from build123d import *

# Parameters (mm, degrees)
SZKIC1_R                         = 14.5
SZKIC1_R_2                       = 5
DODANIE_WYCI_GNI_CIE1_DEPTH      = 15
OTW_R_GWINTOWANY_M61_D           = 5
WYTNIJ_WYCI_GNI_CIE2_DEPTH       = 10
WYTNIJ_WYCI_GNI_CIE4_START       = 20
WYTNIJ_WYCI_GNI_CIE4_DEPTH       = 20
SFAZOWANIE4_SIZE                 = 10
SZKIC17_R                        = 7.5
WYTNIJ_WYCI_GNI_CIE5_DEPTH       = 5
SZKIC17_5_R                      = 7.5
WYTNIJ_WYCI_GNI_CIE6_DEPTH       = 163.311542951
OTW_R_GWINTOWANY_M81_D           = 6.8
OTW_R_GWINTOWANY_M81_DEPTH       = 16.207073895
OTW_R_GWINTOWANY_M81_CSINK_D     = 8.05
OTW_R_GWINTOWANY_M81_CSINK_ANGLE = 90
OTW_R_GWINTOWANY_M81_TIP         = 2.042926105


with BuildPart() as part:
    # Szkic1 → Dodanie-wyci_gni_cie1 (new, symmetric)
    with BuildSketch(Plane(origin=(0, 0, 0), x_dir=(0, 0, -1), z_dir=(1, 0, 0))):
        with BuildLine():
            Line((-72.530533194, -70), (-85.848604083, -57.040111879))
            ThreePointArc((-85.848604083, -57.040111879), (-92.404294481, -44.130927243), (-87.495806927, -30.50995538))
            ThreePointArc((-87.495806927, -30.50995538), (-75.419960244, 0), (-87.495806927, 30.50995538))
            ThreePointArc((-87.495806927, 30.50995538), (-92.32041193, 40.919666146), (-89.978943384, 52.151603499))
            ThreePointArc((-89.978943384, 52.151603499), (-81.115709466, 65.086416999), (-70.408575711, 76.541704099))
            ThreePointArc((-70.408575711, 76.541704099), (-67.080888035, 80.867469231), (-65.40069858, 86.060032436))
            Line((-65.40069858, 86.060032436), (-62.076569761, 109.385977671))
            ThreePointArc((-62.076569761, 109.385977671), (-54.044566654, 124.12820267), (-38.316621209, 130))
            Line((-38.316621209, 130), (38.316621209, 130))
            ThreePointArc((38.316621209, 130), (54.044566654, 124.12820267), (62.076569761, 109.385977671))
            Line((62.076569761, 109.385977671), (65.40069858, 86.060032436))
            ThreePointArc((65.40069858, 86.060032436), (67.080888035, 80.867469231), (70.408575711, 76.541704099))
            ThreePointArc((70.408575711, 76.541704099), (81.115709466, 65.086416999), (89.978943384, 52.151603499))
            ThreePointArc((89.978943384, 52.151603499), (92.32041193, 40.919666146), (87.495806927, 30.50995538))
            ThreePointArc((87.495806927, 30.50995538), (75.419960244, 0), (87.495806927, -30.50995538))
            ThreePointArc((87.495806927, -30.50995538), (92.006314233, -46.663708643), (81.240664282, -59.524081957))
            Line((81.240664282, -59.524081957), (51.469466806, -70))
            Line((51.469466806, -70), (51.469466806, -100))
            ThreePointArc((51.469466806, -100), (48.29757558, -114.988630917), (39.325734007, -127.407407407))
            ThreePointArc((39.325734007, -127.407407407), (36.208235452, -129.329364235), (32.607823953, -130))
            Line((32.607823953, -130), (14.469466806, -130))
            Line((14.469466806, -130), (-35.530533194, -130))
            Line((-35.530533194, -130), (-53.668890342, -130))
            ThreePointArc((-53.668890342, -130), (-57.269301841, -129.329364235), (-60.386800396, -127.407407407))
            ThreePointArc((-60.386800396, -127.407407407), (-69.358641969, -114.988630917), (-72.530533194, -100))
            Line((-72.530533194, -100), (-72.530533194, -70))
        make_face()
        Circle(SZKIC1_R, mode=Mode.SUBTRACT)
        with Locations(Location((74.189369185, -43, 0), (0, 0, 180))):
            Circle(SZKIC1_R_2, mode=Mode.SUBTRACT)
        with Locations(Location((74.189369185, 43, 0), (0, 0, 180))):
            Circle(SZKIC1_R_2, mode=Mode.SUBTRACT)
        with BuildLine():
            Line((14.469466806, -84), (-35.530533194, -84))
            ThreePointArc((-35.530533194, -84), (-51.530533194, -100), (-35.530533194, -116))
            Line((-35.530533194, -116), (14.469466806, -116))
            ThreePointArc((14.469466806, -116), (30.469466806, -100), (14.469466806, -84))
        make_face(mode=Mode.SUBTRACT)
    extrude(amount=DODANIE_WYCI_GNI_CIE1_DEPTH, both=True)

    # Otw_r gwintowany M61 (through all)
    with Locations(Plane(origin=(-15, 0, 0), x_dir=(0, 0, -1), z_dir=(-1, 0, 0))):
        with Locations((-29.434757864, -101.542610293), (50.455604917, -97.355733794)):
            Hole(OTW_R_GWINTOWANY_M61_D / 2)

    # Szkic12 → Wytnij-wyci_gni_cie2 (cut)
    with BuildSketch(Plane(origin=(-15, 0, 0), x_dir=(0, 0, -1), z_dir=(1, 0, 0))):
        with BuildLine():
            Line((28.802174659, 93.483680258), (-9.732880373, 95.503216916))
            ThreePointArc((-9.732880373, 95.503216916), (-14.464348266, 100.758044371), (-9.209520811, 105.489512264))
            Line((-9.209520811, 105.489512264), (29.325534221, 103.469975605))
            ThreePointArc((29.325534221, 103.469975605), (34.057002114, 98.21514815), (28.802174659, 93.483680258))
        make_face()
    extrude(amount=WYTNIJ_WYCI_GNI_CIE2_DEPTH, mode=Mode.SUBTRACT)

    # Szkic16 → Wytnij-wyci_gni_cie4 (cut)
    with BuildSketch(Plane(origin=(-15, 0, 0), x_dir=(0, 0, -1), z_dir=(1, 0, 0)).offset(WYTNIJ_WYCI_GNI_CIE4_START)):
        with BuildLine():
            Line((-53.668890342, -130), (32.607823953, -130))
            ThreePointArc((32.607823953, -130), (36.208235452, -129.329364235), (39.325734007, -127.407407407))
            ThreePointArc((39.325734007, -127.407407407), (48.29757558, -114.988630917), (51.469466806, -100))
            Line((51.469466806, -100), (51.469466806, -70))
            Line((51.469466806, -70), (-72.530533194, -70))
            Line((-72.530533194, -70), (-72.530533194, -100))
            ThreePointArc((-72.530533194, -100), (-69.358641969, -114.988630917), (-60.386800396, -127.407407407))
            ThreePointArc((-60.386800396, -127.407407407), (-57.269301841, -129.329364235), (-53.668890342, -130))
        make_face()
        with BuildLine():
            Line((-35.530533194, -116), (14.469466806, -116))
            ThreePointArc((14.469466806, -116), (30.469466806, -100), (14.469466806, -84))
            Line((14.469466806, -84), (-35.530533194, -84))
            ThreePointArc((-35.530533194, -84), (-51.530533194, -100), (-35.530533194, -116))
        make_face(mode=Mode.SUBTRACT)
    extrude(amount=-WYTNIJ_WYCI_GNI_CIE4_DEPTH, mode=Mode.SUBTRACT)

    # Sfazowanie4
    sfazowanie4_edges = [part.edges().sort_by_distance(p)[0] for p in [
        (-15, -70, 10.530533194),
    ]]
    chamfer(sfazowanie4_edges, length=SFAZOWANIE4_SIZE)

    # Szkic17 → Wytnij-wyci_gni_cie5 (cut)
    with BuildSketch(Plane(origin=(-15, 0, 0), x_dir=(0, 0, -1), z_dir=(1, 0, 0))):
        with BuildLine():
            Line((-45.292857142, 8.957177033), (-31.578571428, 10.93666367))
            ThreePointArc((-31.578571428, 10.93666367), (-22.462605729, 8.080234378), (-18.98012619, -0.815402484))
            ThreePointArc((-18.98012619, -0.815402484), (-23.079412621, -8.614404816), (-31.578571429, -10.936663671))
            Line((-31.578571429, -10.936663671), (-45.292857143, -8.957177034))
            ThreePointArc((-45.292857143, -8.957177034), (-53.05, 0), (-45.292857142, 8.957177033))
        make_face()
        with Locations(Location((-30, -1e-09, 0), (0, 0, 180))):
            Circle(SZKIC17_R, mode=Mode.SUBTRACT)
    extrude(amount=WYTNIJ_WYCI_GNI_CIE5_DEPTH, mode=Mode.SUBTRACT)

    # Szkic17_5 → Wytnij-wyci_gni_cie6 (cut, through all)
    with BuildSketch(Plane(origin=(-15, 0, 0), x_dir=(0, 0, -1), z_dir=(1, 0, 0))):
        with Locations(Location((-30, -1e-09, 0), (0, 0, 180))):
            Circle(SZKIC17_5_R)
    extrude(amount=WYTNIJ_WYCI_GNI_CIE6_DEPTH, mode=Mode.SUBTRACT)

    # Otw_r gwintowany M81
    with Locations(Plane(origin=(5, -77, -39.469466806), x_dir=(0, 0, -1), z_dir=(-1, 0, 0))):
        with Locations((0, 0), (0, 40), (-100, 40), (-100, 0)):
            CounterSinkHole(OTW_R_GWINTOWANY_M81_D / 2, OTW_R_GWINTOWANY_M81_CSINK_D / 2, depth=OTW_R_GWINTOWANY_M81_DEPTH, counter_sink_angle=OTW_R_GWINTOWANY_M81_CSINK_ANGLE)
            with Locations((0, 0, -(OTW_R_GWINTOWANY_M81_DEPTH + OTW_R_GWINTOWANY_M81_TIP / 2))):  # 118° drill point
                Cone(0, OTW_R_GWINTOWANY_M81_D / 2, OTW_R_GWINTOWANY_M81_TIP, mode=Mode.SUBTRACT)


solid = part.part
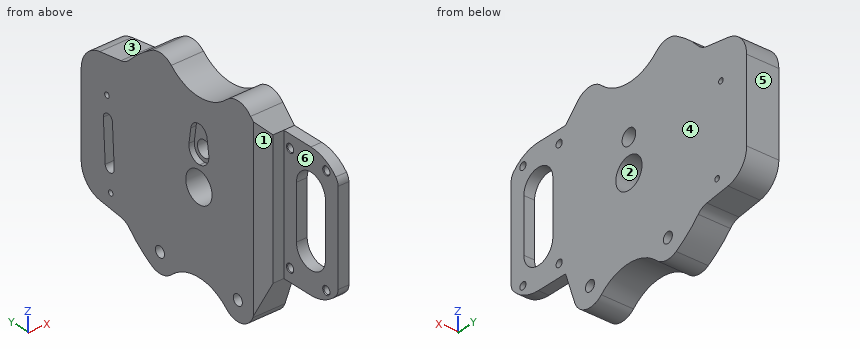
Build history of the part. All positions in model axes, mm. Face numbers are marked on the shaded views. A direction names the side the tool comes from. Round coordinates to 2 decimals unless told otherwise and drop trailing zeros. Loops run counter-clockwise (first coordinate to the right, second up) from the corner with the lowest first, then second, coordinate; pieces in that order, holes last. Notation, with made-up numbers: (83, 60) -> (87, 60) arc R14 cw to (87, 75) -> close; hole circle Ø10 at (76.5, 74). An arc over 180 degrees is marked (long way). One line per item, written item: value. Start each with the question number.
Q1. Two-plate mould, pull along Y, no slides. Class the marked faces 1, 2, 3 and 4: released by +Y, released by -Y, zero draft, split by the parting line, or undercut.
Q2. Cut at A-A on y = -77. List the corners of the cut face in (x, z) (3 decimals), plus the area to 3 significant figures.
Q3. Drop flat-ended pins along their axis: pin 1 Ø1.5 at (x, y) = (-0.5, 76) entering from +Z; pin 2 Ø11 at (y, z) = (-117, -39.47) entering from -X; pin 3 Ø10 at (y, z) = (7, 1) entering from -X; pin 4 Ø6.5 at (y, z) = (-4.5, 40.5) entering from -X. Give the stop position or say it passes through.
Q4. Cut at C-C on x = 2. List the corners of the cut face in (y, z).
Q5. Cut at D-D on z = 42.5. List the corners of the cut face in (x, y), plus the area to 3 significant figures.
Q6. 3-axis set-ups, long thin cutter, end or side, ignore diameter. For the marked faces 5 and 6: which of +Z, -Z, +X, -X, +Y, -Y reach the whole face in a straight line?
Q7. Cut at B-B on z = 0. List the corners of the cut face in (x, y), plus the area to 3 significant figures.
Q8. Probe line 1 along Z through (x, y) = (12.5, -77); line 2 along Y through (x, z) = (-4, 30); line 3 along Y through (x, z) = (-12, -84). List the from-to ranges inside material, lowest first.
Computed:
1. face 1: released by -Y
1. face 2: undercut
1. face 3: released by +Y
1. face 4: zero draft
2. outline: (5, -51.469) -> (15, -51.469) -> (15, -42.869) -> (5.625, -42.869) -> (5, -43.494) -> close; (5, -35.444) -> (5.625, -36.069) -> (15, -36.069) -> (15, 57.131) -> (5.625, 57.131) -> (5, 56.506) -> close; (5, 64.556) -> (5.625, 63.931) -> (15, 63.931) -> (15, 72.531) -> (5, 72.531) -> close
2. area: 1,100 mm²
3. pin 1: z = 71.79
3. pin 2: x = 5
3. pin 3: through
3. pin 4: x = -10
4. outline: (-70, -51.47) -> (-59.52, -81.24) arc R18 ccw to (-30.51, -87.5) arc R44.58 cw to (30.51, -87.5) arc R18.25 ccw to (52.15, -89.98) arc R104 ccw to (76.54, -70.41) arc R16 cw to (86.06, -65.4) -> (109.39, -62.08) arc R24 ccw to (130, -38.32) -> (130, 38.32) arc R24 ccw to (109.39, 62.08) -> (86.06, 65.4) arc R16 cw to (76.54, 70.41) arc R104 ccw to (52.15, 89.98) arc R18.25 ccw to (30.51, 87.5) arc R44.58 cw to (-30.51, 87.5) arc R18.25 ccw to (-57.04, 85.85) -> (-70, 72.53) -> close; hole circle Ø10 at (-43, -74.19); hole circle Ø29 at (0, 0); hole circle Ø15 at (0, 30); hole circle Ø10 at (43, -74.19); hole circle Ø5 at (97.36, -50.46); hole circle Ø5 at (101.54, 29.43)
5. outline: (-15, -60) -> (-5, -70) -> (5, -70) -> (5, -85.6) -> (15, -85.6) -> (15, 129.63) -> (-15, 129.63) -> (-15, 9.36) -> (-10, 9.36) -> (-10, -9.36) -> (-15, -9.36) -> close; (5, -130) -> (15, -130) -> (15, -114.4) -> (5, -114.4) -> close
5. area: 6,160 mm²
6. face 5: +Z, -Z, +X, -X, +Y
6. face 6: +Z, -Z, -X, -Y
7. outline: (-15, -60) -> (-5, -70) -> (5, -70) -> (5, -84) -> (15, -84) -> (15, -14.5) -> (-15, -14.5) -> close; (-15, 14.5) -> (15, 14.5) -> (15, 130) -> (-15, 130) -> (-15, 105.01) -> (-5, 105.01) -> (-5, 94.99) -> (-15, 94.99) -> close; (5, -130) -> (15, -130) -> (15, -116) -> (5, -116) -> close
7. area: 5,260 mm²
8. line 1: -51.47 to -42.87, -36.07 to 57.13, 63.93 to 72.53
8. line 2: -70 to -7.5, 7.5 to 99.11, 103.98 to 130
8. line 3: -58.1 to -26.29, 26.29 to 61.32
